The listing builds one solid part. Answer for the finished solid, in the listing's coordinates (mm). A direction names the side the tool comes from. Give positions to 0.01 mm unless a question says otherwise; leave off trailing zeros. Loops run counter-clockwise (first coordinate to the right, second up) from the corner with the lowest first, then second, coordinate; pieces in that order, holes last.
Item 1: Section C-C, the plane y = -8.5 is taken. Give the vertices of the cut face in (x, z).
Item 2: Each of these flat-tipped pins is pushed along its axis until it touches: pin 1 Ø8 at (x, z) = (0.5, -7) entering from -Y; pin 2 Ø6 at (x, y) = (-3.5, -0.5) entering from +Z; pin 3 Ø6 at (x, y) = (1.5, -10.5) entering from +Z. Where does it stop, or does it pass through?
Item 3: Section A-A, the plane z = -0.75 is taken. Give the vertices of the cut face in (x, y).
Item 4: Section D-D, the plane z = -11.5 is taken. Give the vertices of the cut face in (x, y), and give its area (3 significant figures).
Item 5: The mould has two halves that part along Z. Classify faces 1 (the face through (-0.11, -5.22, -8.53)), 2 (the face through (-0.112, -0.881, -11.045)), 3 (the face through (-0.112, -10.017, -3.255)): pulls with the +Z half, pulls with the -Z half, needs draft (parallel to the pull), parting line crosses it, or undercut.
Item 6: A tool of negligible diameter and unlimited length cuts with its end or side. For faces 4 (the face through (-0.112, 10.017, -3.255)), 5 (the face through (0.112, 3.255, -10.017)), 6 (the face through (-0.11, 1.65, -10.42)), from which of +Z, -Z, +X, -X, +Y, -Y can it reach the whole face along a straight path? Write none if from no direction.
Item 7: Section B-B, the plane y = -2.75 is taken. Give the vertices of the cut face in (x, z).
Item 8: Consider line 1 along Z through (x, y) = (-2.5, -6.25); line 2 along X through (y, z) = (-5.75, -11.5); line 3 along Z through (x, y) = (2.75, 4.75). Determine where each line is inside the solid, lowest interval first.
from build123d import *

# Parameters (mm, degrees)
SKETCH_7_R          = 7
CUT_EXTRUDE_3_DEPTH = 10
CUT_EXTRUDE_4_DEPTH = 8


with BuildPart() as part:
    # 草图1 → 旋转1 (revolve)
    with BuildSketch(Plane.XY):
        Polygon((-9.5, 0), (9.5, 0), (9.5, 13.08), (8, 13.08), (8, 11.08), (-8, 11.08), (-8, 13.08), (-9.5, 13.08), align=None)
    revolve(axis=Axis((-9.5, 0, 0), (1, 0, 0)))

    # 草图7 → 切除-拉伸3 (cut, symmetric)
    with BuildSketch(Plane(origin=(0, 0, 0), x_dir=(0, 0, -1), z_dir=(1, 0, 0))):
        Circle(SKETCH_7_R)
    extrude(amount=CUT_EXTRUDE_3_DEPTH, both=True, mode=Mode.SUBTRACT)

    # 草图2 → 切除-拉伸4 (cut, symmetric)
    with BuildSketch(Plane(origin=(0, 0, 0), x_dir=(0, 0, -1), z_dir=(1, 0, 0))):
        with BuildLine():
            Line((10, 0), (11.08, 0))
            ThreePointArc((11.08, 0), (11.045844058, 0.869326781), (10.943586814, 1.733293873))
            Line((10.943586814, 1.733293873), (9.876883406, 1.56434465))
            ThreePointArc((9.876883406, 1.56434465), (9.969173337, 0.784590957), (10, 0))
        make_face()
        with BuildLine():
            Line((9.510565163, -3.090169944), (10.537706201, -3.423908298))
            ThreePointArc((10.537706201, -3.423908298), (10.773858718, -2.586574632), (10.943586814, -1.733293873))
            Line((10.943586814, -1.733293873), (9.876883406, -1.56434465))
            ThreePointArc((9.876883406, -1.56434465), (9.723699204, -2.334453639), (9.510565163, -3.090169944))
        make_face()
        with BuildLine():
            Line((8.090169944, -5.877852523), (8.963908298, -6.512660595))
            ThreePointArc((8.963908298, -6.512660595), (9.447253021, -5.789284097), (9.872352288, -5.030214737))
            Line((9.872352288, -5.030214737), (8.910065242, -4.539904997))
            ThreePointArc((8.910065242, -4.539904997), (8.526401644, -5.224985647), (8.090169944, -5.877852523))
        make_face()
        with BuildLine():
            Line((5.877852523, -8.090169944), (6.512660595, -8.963908298))
            ThreePointArc((6.512660595, -8.963908298), (7.195884375, -8.425298099), (7.834743136, -7.834743136))
            Line((7.834743136, -7.834743136), (7.071067812, -7.071067812))
            ThreePointArc((7.071067812, -7.071067812), (6.494480483, -7.604059656), (5.877852523, -8.090169944))
        make_face()
        with BuildLine():
            Line((3.090169944, -9.510565163), (3.423908298, -10.537706201))
            ThreePointArc((3.423908298, -10.537706201), (4.240132431, -10.23658522), (5.030214737, -9.872352288))
            Line((5.030214737, -9.872352288), (4.539904997, -8.910065242))
            ThreePointArc((4.539904997, -8.910065242), (3.826834324, -9.238795325), (3.090169944, -9.510565163))
        make_face()
        with BuildLine():
            Line((0, -10), (0, -11.08))
            ThreePointArc((0, -11.08), (0.869326781, -11.045844058), (1.733293873, -10.943586814))
            Line((1.733293873, -10.943586814), (1.56434465, -9.876883406))
            ThreePointArc((1.56434465, -9.876883406), (0.784590957, -9.969173337), (0, -10))
        make_face()
        with BuildLine():
            Line((-3.090169944, -9.510565163), (-3.423908298, -10.537706201))
            ThreePointArc((-3.423908298, -10.537706201), (-2.586574632, -10.773858718), (-1.733293873, -10.943586814))
            Line((-1.733293873, -10.943586814), (-1.56434465, -9.876883406))
            ThreePointArc((-1.56434465, -9.876883406), (-2.334453639, -9.723699204), (-3.090169944, -9.510565163))
        make_face()
        with BuildLine():
            Line((-5.877852523, -8.090169944), (-6.512660595, -8.963908298))
            ThreePointArc((-6.512660595, -8.963908298), (-5.789284097, -9.447253021), (-5.030214737, -9.872352288))
            Line((-5.030214737, -9.872352288), (-4.539904997, -8.910065242))
            ThreePointArc((-4.539904997, -8.910065242), (-5.224985647, -8.526401644), (-5.877852523, -8.090169944))
        make_face()
        with BuildLine():
            Line((-8.090169944, -5.877852523), (-8.963908298, -6.512660595))
            ThreePointArc((-8.963908298, -6.512660595), (-8.425298099, -7.195884375), (-7.834743136, -7.834743136))
            Line((-7.834743136, -7.834743136), (-7.071067812, -7.071067812))
            ThreePointArc((-7.071067812, -7.071067812), (-7.604059656, -6.494480483), (-8.090169944, -5.877852523))
        make_face()
        with BuildLine():
            Line((-9.510565163, -3.090169944), (-10.537706201, -3.423908298))
            ThreePointArc((-10.537706201, -3.423908298), (-10.23658522, -4.240132431), (-9.872352288, -5.030214737))
            Line((-9.872352288, -5.030214737), (-8.910065242, -4.539904997))
            ThreePointArc((-8.910065242, -4.539904997), (-9.238795325, -3.826834324), (-9.510565163, -3.090169944))
        make_face()
        with BuildLine():
            Line((-10, 0), (-11.08, 0))
            ThreePointArc((-11.08, 0), (-11.045844058, -0.869326781), (-10.943586814, -1.733293873))
            Line((-10.943586814, -1.733293873), (-9.876883406, -1.56434465))
            ThreePointArc((-9.876883406, -1.56434465), (-9.969173337, -0.784590957), (-10, 0))
        make_face()
        with BuildLine():
            Line((-9.510565163, 3.090169944), (-10.537706201, 3.423908298))
            ThreePointArc((-10.537706201, 3.423908298), (-10.773858718, 2.586574632), (-10.943586814, 1.733293873))
            Line((-10.943586814, 1.733293873), (-9.876883406, 1.56434465))
            ThreePointArc((-9.876883406, 1.56434465), (-9.723699204, 2.334453639), (-9.510565163, 3.090169944))
        make_face()
        with BuildLine():
            Line((-8.090169944, 5.877852523), (-8.963908298, 6.512660595))
            ThreePointArc((-8.963908298, 6.512660595), (-9.447253021, 5.789284097), (-9.872352288, 5.030214737))
            Line((-9.872352288, 5.030214737), (-8.910065242, 4.539904997))
            ThreePointArc((-8.910065242, 4.539904997), (-8.526401644, 5.224985647), (-8.090169944, 5.877852523))
        make_face()
        with BuildLine():
            Line((-5.877852523, 8.090169944), (-6.512660595, 8.963908298))
            ThreePointArc((-6.512660595, 8.963908298), (-7.195884375, 8.425298099), (-7.834743136, 7.834743136))
            Line((-7.834743136, 7.834743136), (-7.071067812, 7.071067812))
            ThreePointArc((-7.071067812, 7.071067812), (-6.494480483, 7.604059656), (-5.877852523, 8.090169944))
        make_face()
        with BuildLine():
            Line((-3.090169944, 9.510565163), (-3.423908298, 10.537706201))
            ThreePointArc((-3.423908298, 10.537706201), (-4.240132431, 10.23658522), (-5.030214737, 9.872352288))
            Line((-5.030214737, 9.872352288), (-4.539904997, 8.910065242))
            ThreePointArc((-4.539904997, 8.910065242), (-3.826834324, 9.238795325), (-3.090169944, 9.510565163))
        make_face()
        with BuildLine():
            Line((0, 10), (0, 11.08))
            ThreePointArc((0, 11.08), (-0.869326781, 11.045844058), (-1.733293873, 10.943586814))
            Line((-1.733293873, 10.943586814), (-1.56434465, 9.876883406))
            ThreePointArc((-1.56434465, 9.876883406), (-0.784590957, 9.969173337), (0, 10))
        make_face()
        with BuildLine():
            Line((3.090169944, 9.510565163), (3.423908298, 10.537706201))
            ThreePointArc((3.423908298, 10.537706201), (2.586574632, 10.773858718), (1.733293873, 10.943586814))
            Line((1.733293873, 10.943586814), (1.56434465, 9.876883406))
            ThreePointArc((1.56434465, 9.876883406), (2.334453639, 9.723699204), (3.090169944, 9.510565163))
        make_face()
        with BuildLine():
            Line((5.877852523, 8.090169944), (6.512660595, 8.963908298))
            ThreePointArc((6.512660595, 8.963908298), (5.789284097, 9.447253021), (5.030214737, 9.872352288))
            Line((5.030214737, 9.872352288), (4.539904997, 8.910065242))
            ThreePointArc((4.539904997, 8.910065242), (5.224985647, 8.526401644), (5.877852523, 8.090169944))
        make_face()
        with BuildLine():
            Line((8.090169944, 5.877852523), (8.963908298, 6.512660595))
            ThreePointArc((8.963908298, 6.512660595), (8.425298099, 7.195884375), (7.834743136, 7.834743136))
            Line((7.834743136, 7.834743136), (7.071067812, 7.071067812))
            ThreePointArc((7.071067812, 7.071067812), (7.604059656, 6.494480483), (8.090169944, 5.877852523))
        make_face()
        with BuildLine():
            Line((9.510565163, 3.090169944), (10.537706201, 3.423908298))
            ThreePointArc((10.537706201, 3.423908298), (10.23658522, 4.240132431), (9.872352288, 5.030214737))
            Line((9.872352288, 5.030214737), (8.910065242, 4.539904997))
            ThreePointArc((8.910065242, 4.539904997), (9.238795325, 3.826834324), (9.510565163, 3.090169944))
        make_face()
    extrude(amount=CUT_EXTRUDE_4_DEPTH, both=True, mode=Mode.SUBTRACT)


solid = part.part
Worked answers:
1. outline: (-9.5, -9.94) - (-8, -9.94) - (-8, -6.18) - (8, -6.18) - (8, -9.94) - (9.5, -9.94) - (9.5, 9.94) - (8, 9.94) - (8, 7.11) - (-8, 7.11) - (-8, 9.94) - (-9.5, 9.94) - close; hole (-8, 5.27) - (8, 5.27) - (8, 6.18) - (-8, 6.18) - close
2. pin 1: stops at y = -10.67
2. pin 2: stops at z = 11.08
2. pin 3: stops at z = 7.83
3. outline: (-9.5, -13.06) - (-8, -13.06) - (-8, -9.97) - (8, -9.97) - (8, -13.06) - (9.5, -13.06) - (9.5, -6.96) - (-9.5, -6.96) - close; (-9.5, 6.96) - (9.5, 6.96) - (9.5, 13.06) - (8, 13.06) - (8, 11.05) - (-8, 11.05) - (-8, 13.06) - (-9.5, 13.06) - close
4. outline: (-9.5, -6.23) - (-8, -6.23) - (-8, 6.23) - (-9.5, 6.23) - close; (8, -6.23) - (9.5, -6.23) - (9.5, 6.23) - (8, 6.23) - close
4. area: 37.4 mm2
5. face 1: undercut
5. face 2: pulls with the -Z half
5. face 3: undercut
6. face 4: +Y
6. face 5: none
6. face 6: -Z
7. outline: (-9.5, -12.79) - (-8, -12.79) - (-8, -9.61) - (8, -9.61) - (8, -12.79) - (9.5, -12.79) - (9.5, -6.44) - (-9.5, -6.44) - close; (-9.5, 6.44) - (9.5, 6.44) - (9.5, 12.79) - (8, 12.79) - (8, 10.73) - (-8, 10.73) - (-8, 12.79) - (-9.5, 12.79) - close
8. line 1: z = -8.6 to -3.15, 3.15 to 7.81, 8.6 to 9.15
8. line 2: x = -9.5 to -8, 8 to 9.5
8. line 3: z = -9.32 to -5.14, 5.14 to 8.8, 9.32 to 10.01
